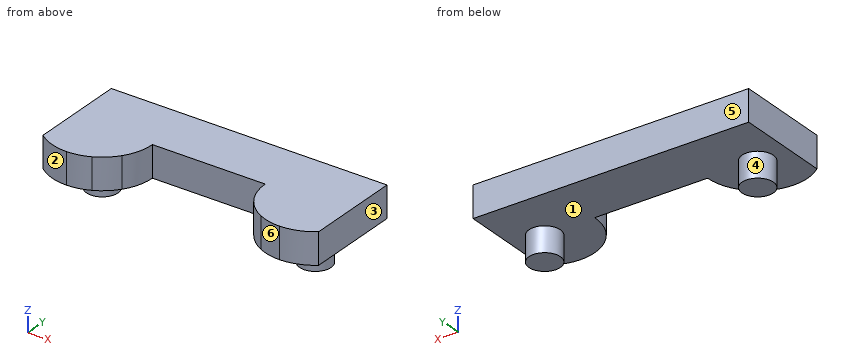
Autodesk Inventor part; units mm, degrees
ref_plane "作業平面1" through (-20, -16, -4) normal (0, 0, 1) x (1, 0, 0)
ref_plane "YZ Plane" through (0, 0, 0) normal (1, 0, 0) x (0, 1, 0)
ref_plane "XZ Plane" through (0, 0, 0) normal (0, 1, 0) x (-1, 0, 0)
sketch "スケッチ1" plane through (0, 0, 0) normal (0, 0, 1) x (1, 0, 0)
  line L0 (-22, 30) -> (22, 30)
  line L1 (22, 30) -> (22, 0)
  line L2 (22, 0) -> (-22, 0)
  line L3 (-22, 0) -> (-22, 30)
  point P0 (0, 0)
  point P1 (0, 0)
  dimension "d0" = 30
  dimension "d1" = 44
extrude "押し出し1" add sketch "スケッチ1" along normal blind 5
sketch "スケッチ2" plane through (0, 0, 5) normal (0, 0, 1) x (1, 0, 0)
  arc A0 (-17, 13) -> (-13.5, 13.8063) centre (-17, 21) ccw
  arc A1 (-10.5, 16.3363) -> (-9, 21) centre (-17, 21) ccw
  line L0 (-7.5, 21) -> (-9, 21)
  line L1 (-1.5, 21) -> (-4.5, 21)
  arc A2 (9, 21) -> (10.5, 16.3363) centre (17, 21) ccw
  arc A3 (13.5, 13.8063) -> (17, 13) centre (17, 21) ccw
  circle A4 centre (-17, 21) radius 8
  circle A5 centre (17, 21) radius 8
  line L2 (-9, 21) -> (9, 21)
  line L3 (-22, 0) -> (22, 0)
  line L4 (22, 0) -> (22, 30)
  line L5 (22, 30) -> (-22, 30)
  line L6 (-22, 30) -> (-22, 0)
  point P0 (0, 0)
  point P1 (22, 14.755)
  point P2 (17, 13)
  point P3 (10.5, 16.3363)
  point P4 (-13.5, 13.8063)
  point P5 (-17, 13)
  point P6 (-22, 14.755)
extrude "押し出し2" cut sketch "スケッチ2" against normal through all contours A0 A4 A1 L0 L2 L1 A2 A5 A3 L4 L3 L6
sketch "スケッチ3" plane through (0, 0, 0) normal (0, 0, -1) x (-1, 0, 0)
  circle A0 centre (-17, 21) radius 3
  circle A1 centre (17, 21) radius 3
  circle A2 centre (-17, 21) radius 2.5
  circle A3 centre (17, 21) radius 2.5
  point P0 (0, 0)
  point P1 (-14.9, 18.325)
  dimension "d6" = 5
  dimension "d7" = 5
ref_plane "作業平面1" through (-20, -16, -4) normal (0, 0, 1) x (1, 0, 0)
extrude "押し出し3" add sketch "スケッチ3" along normal up to surface (4 mm away) contours A2 | A3
properties part number "board_setter_upper"
Source: CAD feature listing. Evaluate the final solid. Frame: model axes, mm. Face numbers are marked on the shaded views. A direction names the side the tool comes from. Give positions to 0.01 mm unless a question says otherwise; leave off trailing zeros. Loops run counter-clockwise (first coordinate to the right, second up) from the corner with the lowest first, then second, coordinate; pieces in that order, holes last. Notation, with made-up numbers: (44.25, -30.5) -> (48.25, -30.5) arc R10 cw to (48.25, -23.5) -> close; hole circle Ø5 at (13, -13.75). An arc over 180 degrees is marked (long way). Use a Markdown table: item, result. Add a question column.
(1) Section query B-B (z = -0.5). Output: boundary loops of the cut face in (x, y).
(2) Section query D-D (z = 3). Output: boundary loops of the cut face in (x, y) (3 decimals).
(3) First-contact query: pin 1 Ø2 at (x, y) = (-3.5, 26.5) entering from -Z; pin 2 Ø1 at (x, z) = (11.5, -1.5) entering from -Y; pin 3 Ø2 at (x, z) = (-13, 1.5) entering from -Y; pin 4 Ø2.5 at (x, z) = (-3, 1.5) entering from -Y. Flat tips, straight axial feed; report the tip coordinate or a pass-through.
(4) Pull-direction query (X, two-part tool) for the marked faces 1, 2 and 3; classes: +X half, -X half, draft (parallel to the pull), parting line (faces both ways), or undercut.
(5) Ray query, line 1 (Z direction, x = -13, y = 28.5); line 2 (Y direction, x = -5, z = 0.5); line 3 (X direction, y = 22, z = -1). Return the intervals inside material, ascending.
(6) Section query A-A (y = 15.25). Output: boundary loops of the cut face in (x, z), then the cut area to 3 significant figures.
(7) Access query for the marked faces 4, 5 and 6. Directions: +Z, -Z, +X, -X, +Y, -Y. A direction counts if a zero-diameter tool reaches every point of the face in a straight line with its end or side. Return the directions, or none.
(8) Section query C-C (x = -7.5). Output: boundary loops of the cut face in (y, z).
Checked values:
| question | item | result |
|---|---|---|
| 1 | outline | circle Ø5 at (-17, 21); circle Ø5 at (17, 21) |
| 2 | outline | (-22, 14.755) arc R8 ccw to (-17, 13) arc R7.999 ccw to (-13.5, 13.806) arc R8 ccw to (-10.5, 16.336) arc R8 ccw to (-9, 21) -> (9, 21) arc R8 ccw to (10.5, 16.336) arc R8 ccw to (13.5, 13.806) arc R8.001 ccw to (17, 13) arc R8 ccw to (22, 14.755) -> (22, 30) -> (-22, 30) -> close |
| 3 | pin 1 | z = 0 |
| 3 | pin 2 | through |
| 3 | pin 3 | y = 13.58 |
| 3 | pin 4 | y = 21 |
| 4 | face 1 | undercut |
| 4 | face 2 | -X half |
| 4 | face 3 | +X half |
| 5 | line 1 | 0 to 5 |
| 5 | line 2 | 21 to 30 |
| 5 | line 3 | -19.29 to -14.71, 14.71 to 19.29 |
| 6 | outline | (-22, 0) -> (-11.44, 0) -> (-11.44, 5) -> (-22, 5) -> close; (11.44, 0) -> (22, 0) -> (22, 5) -> (11.44, 5) -> close |
| 6 | area | 106 mm^2 |
| 7 | face 4 | -Z |
| 7 | face 5 | +Z, -Z, +X, -X, +Y |
| 7 | face 6 | +Z, -Z, -Y |
| 8 | outline | (21, 0) -> (30, 0) -> (30, 5) -> (21, 5) -> close |
